from build123d import *

# Parameters (mm, degrees)
SKETCH1_W           = 31.6
SKETCH1_H           = 31.6
SKETCH1_W_2         = 25.6
SKETCH1_H_2         = 25.6
BOSS_EXTRUDE1_DEPTH = 35
SKETCH2_W           = 4.5
SKETCH2_H           = 31.6
BOSS_EXTRUDE2_DEPTH = 70.5
FILLET1_R           = 10
SKETCH3_W           = 11.8
SKETCH3_H           = 60.5
CUT_EXTRUDE1_DEPTH  = 13
FILLET2_R           = 10
FILLET3_R           = 4
FILLET4_R           = 4
FILLET5_R           = 4
FILLET6_R           = 4
SKETCH4_R           = 3.43
CUT_EXTRUDE2_DEPTH  = 13
SKETCH6_W           = 4.5
SKETCH6_H           = 25.6
BOSS_EXTRUDE3_DEPTH = 26


# Some blends are built 0.0001 mm under size
with BuildPart() as part:
    # Sketch1 → Boss-Extrude1 (new body)
    with BuildSketch(Plane(origin=(0, 0, 0), x_dir=(0, 0, -1), z_dir=(1, 0, 0))):
        Rectangle(SKETCH1_W, SKETCH1_H)
        Rectangle(SKETCH1_W_2, SKETCH1_H_2, mode=Mode.SUBTRACT)
    extrude(amount=BOSS_EXTRUDE1_DEPTH)

    # Sketch2 → Boss-Extrude2 (add)
    with BuildSketch(Plane(origin=(0, 15.8, 0), x_dir=(1, 0, 0), z_dir=(0, 1, 0))):
        with Locations((2.25, 0)):
            Rectangle(SKETCH2_W, SKETCH2_H)
    extrude(amount=BOSS_EXTRUDE2_DEPTH)

    # Fillet1
    fillet1_edges = [part.edges().sort_by_distance(p)[0] for p in [
        (4.5, 15.8, 0),
    ]]
    fillet(fillet1_edges, radius=FILLET1_R)

    # Sketch3 → Cut-Extrude1 (cut)
    with BuildSketch(Plane(origin=(4.5, 0, 0), x_dir=(0, 0, -1), z_dir=(1, 0, 0))):
        with BuildLine():
            Line((-2, 45.8), (-2, 47.8))
            ThreePointArc((-2, 47.8), (0, 49.8), (2, 47.8))
            Line((2, 47.8), (2, 45.8))
            ThreePointArc((2, 45.8), (0, 43.8), (-2, 45.8))
        make_face()
        with BuildLine():
            Line((-2, 60.3), (-2, 62.3))
            ThreePointArc((-2, 62.3), (0, 64.3), (2, 62.3))
            Line((2, 62.3), (2, 60.3))
            ThreePointArc((2, 60.3), (0, 58.3), (-2, 60.3))
        make_face()
        with BuildLine():
            Line((-2, 78.3), (-2, 80.3))
            ThreePointArc((-2, 80.3), (0, 82.3), (2, 80.3))
            Line((2, 80.3), (2, 78.3))
            ThreePointArc((2, 78.3), (0, 76.3), (-2, 78.3))
        make_face()
        with Locations((-9.9, 56.05)):
            Rectangle(SKETCH3_W, SKETCH3_H)
        with Locations((9.9, 56.05)):
            Rectangle(SKETCH3_W, SKETCH3_H)
    extrude(amount=-CUT_EXTRUDE1_DEPTH, mode=Mode.SUBTRACT)

    # Fillet2
    fillet2_edges = [part.edges().sort_by_distance(p)[0] for p in [
        (2.25, 25.8, 4),
        (2.25, 25.8, -4),
    ]]
    fillet(fillet2_edges, radius=FILLET2_R)

    # Fillet3
    fillet3_edges = [part.edges().sort_by_distance(p)[0] for p in [
        (2.25, 86.3, 4),
    ]]
    fillet(fillet3_edges, radius=FILLET3_R)

    # Fillet4
    fillet4_edges = [part.edges().sort_by_distance(p)[0] for p in [
        (2.25, 86.3, -4),
    ]]
    fillet(fillet4_edges, radius=FILLET4_R - 0.0001)  # a hair under: the kernel refuses the full size

    # Fillet5
    # the kernel refuses this fillet: 4 mm, written as the material it takes off along each edge
    with BuildSketch(Plane(origin=(14.065155865, 25.8, 15.8), x_dir=(0, 0.03682620114116805, -0.9993216853994064), z_dir=(-1, 0, 0))) as fillet5_piece_1:
        with BuildLine():
            CenterArc((3.8563874, 3.970771877), FILLET5_R, 182.110463108, 80.958903851)
            Line((-0.140899342, 3.823467072), (-0.540628016, 3.808736592))
            Line((-0.540628016, 3.808736592), (-0.399728674, -0.01473048))
            Line((-0.399728674, -0.01473048), (0.01473048, -0.399728674))
            ThreePointArc((0.01473048, -0.399728674), (1.813509514, -0.333441512), (3.325449974, -0.397077188))
            Line((3.325449974, -0.397077188), (3.373717013, 0))
        make_face()
    extrude(amount=23.630311731, mode=Mode.SUBTRACT)

    # Fillet6
    # the kernel refuses this fillet: 4 mm, written as the material it takes off along each edge
    with BuildSketch(Plane(origin=(14.065155865, 25.8, -15.8), x_dir=(0, 0.03682620114116807, 0.9993216853994065), z_dir=(-1, 0, 0))) as fillet6_piece_1:
        with BuildLine():
            CenterArc((3.8563874, -3.970771877), FILLET6_R, 96.93063304, 80.958903851)
            Line((-0.140899342, -3.823467072), (-0.540628016, -3.808736592))
            Line((-0.540628016, -3.808736592), (-0.399728674, 0.01473048))
            Line((-0.399728674, 0.01473048), (0.01473048, 0.399728674))
            ThreePointArc((0.01473048, 0.399728674), (1.813509514, 0.333441512), (3.325449974, 0.397077188))
            Line((3.325449974, 0.397077188), (3.373717013, 0))
        make_face()
    extrude(amount=23.630311731, mode=Mode.SUBTRACT)

    # Sketch4 → Cut-Extrude2 (cut)
    with BuildSketch(Plane(origin=(0, 15.8, 0), x_dir=(1, 0, 0), z_dir=(0, 1, 0))):
        with Locations(Location((24.75, 0, 0), (0, 0, 270))):
            Circle(SKETCH4_R)
    extrude(amount=-CUT_EXTRUDE2_DEPTH, mode=Mode.SUBTRACT)

    # Sketch6 → Boss-Extrude3 (add)
    with BuildSketch(Plane(origin=(0, -12.8, 0), x_dir=(1, 0, 0), z_dir=(0, 1, 0))):
        with Locations((2.25, 0)):
            Rectangle(SKETCH6_W, SKETCH6_H)
    extrude(amount=BOSS_EXTRUDE3_DEPTH)


solid = part.part
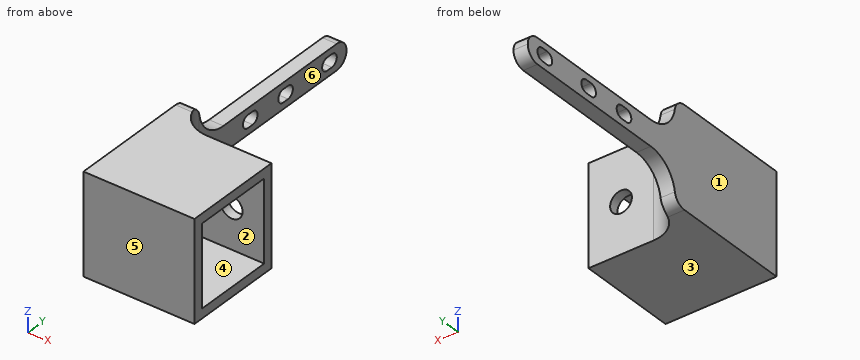
Input: part model. Units: mm. Frame: model coordinates. Face numbers are marked on the shaded views. A direction names the side the tool comes from. Give positions to 0.01 mm unless a question says otherwise; leave off trailing zeros. Order: outer loops, then holes, each group sorted by start corner. A loop starts at its lowest first (then second) coordinate and runs counter-clockwise, first axis right, second up. Notation, with made-up numbers: M -14,18.25 L 12,18.25 A11 ccw 12,32.25 Z; hole C -9,-14.75 d6. An arc over 180 degrees is marked long. Answer as a JSON object with one key per item and string values.
1. Ray query, line 1 (X direction, y = 15, z = 0); line 2 (Y direction, x = 33, z = 5). Return the intervals inside material, ascending. Write a range as [from, to].
Result sheet:
{"line 1": "[0, 21.32], [28.18, 35]", "line 2": "[-15.8, -12.8], [12.8, 15.8]"}
2. Cut plane D-D, the plane z = -5. Output: boundary loops of the cut face in (x, y), and give its area (3 significant figures).
Result sheet:
{"outline": "M 0,-15.8 L 35,-15.8 L 35,-12.8 L 4.5,-12.8 L 4.5,12.8 L 35,12.8 L 35,15.8 L 14.5,15.8 A10 cw 4.5,25.8 L 4.5,31.44 L 0,31.44 Z", "area": "417 mm²"}
3. Reachability of the marked faces 5 and 6 from +Z, -Z, +X, -X, +Y, -Y: full face, straight path, thin tool, end or side. Return the list, or none.
Result sheet:
{"face 5": "+Z, -Z, +X, -X, -Y", "face 6": "+Z, -Z, +X, +Y"}
4. Cut plane C-C, the plane y = 72.5. Output: boundary loops of the cut face in (x, z), and give its area (3 significant figures).
Result sheet:
{"outline": "M 0,-4 L 4.5,-4 L 4.5,4 L 0,4 Z", "area": "36.0 mm²"}
5. Cut plane B-B, the plane x = 24.75. Output: boundary loops of the cut face in (y, z).
Result sheet:
{"outline": "M -15.8,-15.8 L 15.8,-15.8 L 15.8,-3.43 L 12.8,-3.43 L 12.8,-12.8 L -12.8,-12.8 L -12.8,12.8 L 12.8,12.8 L 12.8,3.43 L 15.8,3.43 L 15.8,15.8 L -15.8,15.8 Z"}
6. Cut plane A-A, the plane x = 12.5. Output: boundary loops of the cut face in (y, z), and give its area (3 significant figures).
Result sheet:
{"outline": "M -15.8,-15.8 L 16,-15.8 L 16,15.8 L -15.8,15.8 Z; hole M -12.8,-12.8 L 12.8,-12.8 L 12.8,12.8 L -12.8,12.8 Z", "area": "350 mm²"}
7. First-contact query: P1, Ø0.6, axis at x = 3, y = 61.5, coming from the +Z side; P2, Ø6, axis at x = 28, z = 3, coming from the +Y side; P3, Ø1, axis at x = 1.5, y = 61.5, coming from the -Z side; P4, Ø2, axis at x = 14.5, y = 16.5, coming from the +Z side. Flat tips, straight axial feed; report the tip coordinate or a pass-through.
Result sheet:
{"P1": "z = 4", "P2": "y = 15.8", "P3": "z = -4", "P4": "z = 15.8"}
8. Pull-direction query (Z, two-part tool) for the marked faces 1, 2, 3 and 4; classes: +Z half, -Z half, draft (parallel to the pull), parting line (faces both ways), or undercut.
Result sheet:
{"face 1": "draft", "face 2": "undercut", "face 3": "-Z half", "face 4": "undercut"}
